Design review of the part built by this model. Coordinates are the model's own, in mm. A direction names the side the tool comes from. Coordinates: 2 decimals unless noted, no trailing zeros. Loops run counter-clockwise (first coordinate to the right, second up) from the corner with the lowest first, then second, coordinate; pieces in that order, holes last.
Q1. Add section A-A on x = 35.5. Give the boundary of the cut face in (y, z).
Q2. Add section C-C on y = 19.25. Give the boundary of the cut face in (x, z).
Q3. Add section D-D on x = -1. Give the boundary of the cut face in (y, z).
Q4. Draft analysis for pull direction X (two halves, no side actions). For faces 1 (the face through (45, 1, 0)), 2 (the face through (26, 1, -17.75)), 3 (the face through (-40, 23, 26)), state which applies: released by +X, released by -X, zero draft, split by the parting line, or undercut.
Q5. Machinability: for faces 4 (the face through (18, 23, -23)), 5 (the face through (37, 1, 6.75)), which of the approach directions +Z, -Z, +X, -X, +Y, -Y give a long, thin tool a straight path to every point of the face, cutting with its end or side? Answer none if there is none.
Q6. Add section B-B on z = -24.5. Give the boundary of the cut face in (x, y).
Q7. Wall thickness on probe 1 along X at (y, z) = (12.25, 24.5); probe 2 along Y at (x, z) = (33, 29); probe 3 along Z at (x, y) = (17, 11.75): over which ranges is each line inside the solid? List them lowest first.
Q8. For P1, Ø10, axis at y = 18.5, z = 23, coming from the -X side; P2, Ø10, axis at y = 7.5, z = -16, coming from the -X side; P3, Ø12, axis at x = -36, y = 13, coming from the -Z side, all flat-tipped, find the tip position at first contact; note any pin that passes through.
```python
from build123d import *

# Parameters (mm, degrees)
SKIZZE1_W                       = 90
SKIZZE1_H                       = 65
AUFSATZ_LINEAR_AUSTRAGEN1_DEPTH = 3
SKIZZE3_R                       = 2.5
AUFSATZ_LINEAR_AUSTRAGEN2_DEPTH = 20
SKIZZE4_R                       = 1.364499713
SCHNITT_LINEAR_AUSTRAGEN2_DEPTH = 61.085355953
VERRUNDUNG1_R                   = 3
VERRUNDUNG2_R                   = 1
SKIZZE5_R                       = 12.500347999
SCHNITT_LINEAR_AUSTRAGEN3_DEPTH = 61.085355953
SKIZZE6_W                       = 7
SKIZZE6_H                       = 1.5
SCHNITT_LINEAR_AUSTRAGEN4_DEPTH = 61.085355953
LINEARES_MUSTER1_COUNT          = 4
LINEARES_MUSTER1_PITCH          = 13


with BuildPart() as part:
    # Skizze1 → Aufsatz-Linear austragen1 (new body)
    with BuildSketch(Plane(origin=(0, 0, 0), x_dir=(1, 0, 0), z_dir=(0, 1, 0))):
        Rectangle(SKIZZE1_W, SKIZZE1_H)
    extrude(amount=AUFSATZ_LINEAR_AUSTRAGEN1_DEPTH)

    # Skizze3 → Aufsatz-Linear austragen2 (add)
    with BuildSketch(Plane(origin=(0, 3, 0), x_dir=(1, 0, 0), z_dir=(0, 1, 0))):
        with Locations(Location((-39, 24.5, 0), (0, 0, 270))):
            Circle(SKIZZE3_R)
        with Locations(Location((19.085512482, 24.5, 0), (0, 0, 270))):
            Circle(SKIZZE3_R)
        with Locations(Location((19.085512482, -24.5, 0), (0, 0, 270))):
            Circle(SKIZZE3_R)
        with Locations(Location((-39, -24.5, 0), (0, 0, 270))):
            Circle(SKIZZE3_R)
    extrude(amount=AUFSATZ_LINEAR_AUSTRAGEN2_DEPTH)

    # Skizze4 → Schnitt-Linear austragen2 (cut, through all)
    with BuildSketch(Plane(origin=(0, 23, 0), x_dir=(1, 0, 0), z_dir=(0, 1, 0))):
        with Locations(Location((19.085512482, 24.5, 0), (0, 0, 270))):
            Circle(SKIZZE4_R)
        with Locations(Location((-39, 24.5, 0), (0, 0, 270))):
            Circle(SKIZZE4_R)
        with Locations(Location((-39, -24.5, 0), (0, 0, 270))):
            Circle(SKIZZE4_R)
        with Locations(Location((19.085512482, -24.5, 0), (0, 0, 270))):
            Circle(SKIZZE4_R)
    extrude(amount=-SCHNITT_LINEAR_AUSTRAGEN2_DEPTH, mode=Mode.SUBTRACT)

    # Verrundung1
    verrundung1_edges = [part.edges().sort_by_distance(p)[0] for p in [
        (-45, 1.5, 32.5),
        (-45, 1.5, -32.5),
        (45, 1.5, -32.5),
        (45, 1.5, 32.5),
    ]]
    fillet(verrundung1_edges, radius=VERRUNDUNG1_R)

    # Verrundung2
    verrundung2_edges = [part.edges().sort_by_distance(p)[0] for p in [
        (-39, 3, -27),
        (19.085512482, 3, -27),
        (19.085512482, 3, 22),
        (-39, 3, 22),
    ]]
    fillet(verrundung2_edges, radius=VERRUNDUNG2_R)

    # Skizze5 → Schnitt-Linear austragen3 (cut, through all)
    with BuildSketch(Plane.XZ):
        with Locations(Location((-1, 6.5, 0), (0, 0, 270))):
            Circle(SKIZZE5_R)
    extrude(amount=-SCHNITT_LINEAR_AUSTRAGEN3_DEPTH, mode=Mode.SUBTRACT)

    # Skizze6 → Schnitt-Linear austragen4 (cut, through all)
    with BuildSketch(Plane.XZ):
        with Locations((-37, 20.5)):
            Rectangle(SKIZZE6_W, SKIZZE6_H)
        with Locations((-26, 20.5)):
            Rectangle(SKIZZE6_W, SKIZZE6_H)
        with Locations((26, 20.5)):
            Rectangle(SKIZZE6_W, SKIZZE6_H)
        with Locations((37, 20.5)):
            Rectangle(SKIZZE6_W, SKIZZE6_H)
    schnitt_linear_austragen4 = extrude(amount=-SCHNITT_LINEAR_AUSTRAGEN4_DEPTH, mode=Mode.SUBTRACT)

    # Lineares Muster1: Schnitt-Linear austragen4 ×4
    with Locations(*[(0, 0, -i * LINEARES_MUSTER1_PITCH) for i in range(1, LINEARES_MUSTER1_COUNT)]):
        add(schnitt_linear_austragen4, mode=Mode.SUBTRACT)


solid = part.part
```
Entries:
1. outline: (0, -32.5) - (3, -32.5) - (3, -19.25) - (0, -19.25) - close; (0, -17.75) - (3, -17.75) - (3, -6.25) - (0, -6.25) - close; (0, -4.75) - (3, -4.75) - (3, 6.75) - (0, 6.75) - close; (0, 8.25) - (3, 8.25) - (3, 19.75) - (0, 19.75) - close; (0, 21.25) - (3, 21.25) - (3, 32.5) - (0, 32.5) - close
2. outline: circle Ø5 at (-39, -24.5); circle Ø5 at (-39, 24.5); circle Ø5 at (19.09, -24.5); circle Ø5 at (19.09, 24.5); hole circle Ø2.73 at (-39, -24.5); hole circle Ø2.73 at (-39, 24.5); hole circle Ø2.73 at (19.09, -24.5); hole circle Ø2.73 at (19.09, 24.5)
3. outline: (0, -32.5) - (3, -32.5) - (3, -6) - (0, -6) - close; (0, 19) - (3, 19) - (3, 32.5) - (0, 32.5) - close
4. face 1: released by +X
4. face 2: undercut
4. face 3: zero draft
5. face 4: +Z, -Z, +X, -X, +Y
5. face 5: +Y, -Y
6. outline: (-45, 0) - (-40.36, 0) - (-40.36, 23) - (-41.5, 23) - (-41.5, 4) arc R1 cw to (-42.5, 3) - (-45, 3) - close; (-37.64, 0) - (17.72, 0) - (17.72, 23) - (16.59, 23) - (16.59, 4) arc R1 cw to (15.59, 3) - (-35.5, 3) arc R1 cw to (-36.5, 4) - (-36.5, 23) - (-37.64, 23) - close; (20.45, 0) - (45, 0) - (45, 3) - (22.59, 3) arc R1 cw to (21.59, 4) - (21.59, 23) - (20.45, 23) - close
7. probe 1: x = -41.5 to -40.36, -37.64 to -36.5, 16.59 to 17.72, 20.45 to 21.59
7. probe 2: y = 0 to 3
7. probe 3: z = -25.88 to -23.12, 23.12 to 25.88
8. P1: stops at x = -41.5
8. P2: stops at x = -45
8. P3: stops at z = -27
